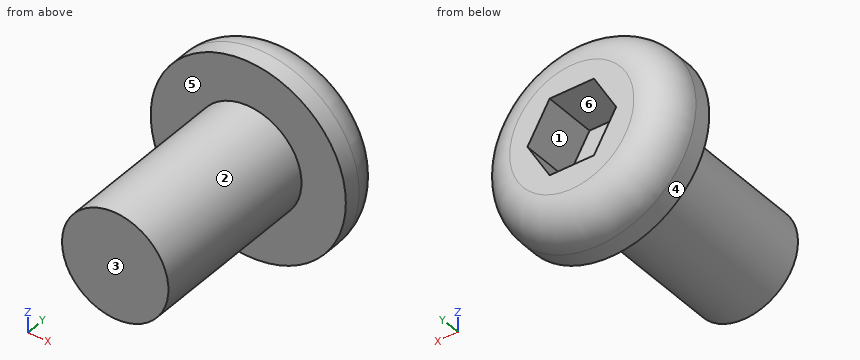
Autodesk Inventor part; units mm, degrees
ref_plane "YZ Plane" through (0, 0, 0) normal (1, 0, 0) x (0, 1, 0)
ref_plane "XZ Plane" through (0, 0, 0) normal (0, 1, 0) x (-1, 0, 0)
ref_plane "XY Plane" through (0, 0, 0) normal (0, 0, 1) x (1, 0, 0)
sketch "Sketch1" plane through (0, 0, 0) normal (0, 1, 0) x (-1, 0, 0)
  circle A0 centre (0, 0) radius 1.5
  dimension "d0" = 3
extrude "Extrusion1" add sketch "Sketch1" along normal blind 5
sketch "Sketch2" plane through (0, 5, 0) normal (0, 1, 0) x (1, 0, 0)
  circle A0 centre (0, 0) radius 1.25 construction
  line L0 (-1.25, 0) -> (-0.625, 1.0825)
  line L1 (-0.625, 1.0825) -> (0.625, 1.0825)
  line L2 (0.625, 1.0825) -> (1.25, 0)
  line L3 (1.25, 0) -> (0.625, -1.0825)
  line L4 (0.625, -1.0825) -> (-0.625, -1.0825)
  line L5 (-0.625, -1.0825) -> (-1.25, 0)
  circle A1 centre (0, 0) radius 2.75
  dimension "d3" = 2.5
  dimension "d4" = 5.5
extrude "Extrusion2" add sketch "Sketch2" along normal blind 1.5
fillet "Fillet1" radius 1 1 edges at (-2.75, 6.5, 0)
thread "Thread1"
properties part number "4mmScrew"
Verification items for the finished model (mm, model axes). Face numbers are marked on the shaded views. A direction names the side the tool comes from. Give positions to 0.01 mm unless a question says otherwise; leave off trailing zeros. Loops run counter-clockwise (first coordinate to the right, second up) from the corner with the lowest first, then second, coordinate; pieces in that order, holes last. Notation, with made-up numbers: M 3.25,83 L 58.25,83 A21 ccw 58.25,101 Z; hole C -14,9 d6. An arc over 180 degrees is marked long. Return JSON: item names as keys, results as strings.
1) Section check A-A, the plane x = 0. Enter the section's corners in (y, z).
Findings:
{"outline": "M 0,-1.5 L 5,-1.5 L 5,-2.75 L 5.5,-2.75 A1 ccw 6.5,-1.75 L 6.5,-1.08 L 5,-1.08 L 5,1.08 L 6.5,1.08 L 6.5,1.75 A1 ccw 5.5,2.75 L 5,2.75 L 5,1.5 L 0,1.5 Z"}
2) Mould release check, pull along X, two halves, no side actions. Record for the marked faces 4, 5 and 6: released by +X, released by -X, zero draft, split by the parting line, or undercut.
Findings:
{"face 4": "split by the parting line", "face 5": "zero draft", "face 6": "undercut"}
3) Tool access check on the marked faces 1, 2 and 3. Record the directions out of +Z, -Z, +X, -X, +Y, -Y that give a thin tool (end or side, any length) a straight path to the whole face; none if there is none.
Findings:
{"face 1": "+Y", "face 2": "-Y", "face 3": "+Z, -Z, +X, -X, -Y"}
4) Material ranges on L1, parallel to Z at x = 0.35, y = 6; L2, parallel to Z at x = -0.6, y = 6.25; L3, parallel to Z at x = -0.05, y = 3.25, recorded low to high. Write a range as [from, to].
Findings:
{"L1": "z = [-2.59, -1.08], [1.08, 2.59]", "L2": "z = [-2.34, -1.08], [1.08, 2.34]", "L3": "z = [-1.5, 1.5]"}
5) Gauge pin test, flat ends, axial feed: P1, Ø2, axis at x = -1, y = 3, coming from the -Z side; P2, Ø0.6, axis at x = -0.5, z = 0, coming from the +Y side; P3, Ø0.6, axis at x = 0, y = 6, coming from the -Z side. Record the tip position at first contact, or that the pin passes through.
Findings:
{"P1": "stops at z = -1.5", "P2": "stops at y = 5", "P3": "stops at z = -2.73"}
